Geometry check sheet. Reference: the model listing, model coordinates, mm. A direction names the side the tool comes from. Round coordinates to 2 decimals unless told otherwise and drop trailing zeros. Write each loop counter-clockwise with the first axis right and the second up, starting at its lowest first coordinate (ties: lowest second). Pieces come first, ordered by that corner, then holes. Notation, with made-up numbers: (-13.75, 58) -> (1.25, 58) arc R26 cw to (1.25, 81) -> close; hole circle Ø2 at (29, -35.5). An arc over 180 degrees is marked (long way). One line per question, with ' | ' between items.
Solid Edge part; units mm, degrees
sketch "Sketch1" plane through (0, 0, 0) normal (0, -1, 0) x (1, 0, 0)
  circle A0 centre (-17.5, 0) radius 1.6
  line L0 (-20.75, -18.3456) -> (-20.75, 0)
  line L1 (-9, -18.3456) -> (-20.75, -18.3456)
  line L2 (-9, -11.0482) -> (-9, -18.3456)
  arc A1 (-14.25, 0) -> (-9, -11.0482) centre (0, 0) ccw
  arc A2 (-20.75, 0) -> (-14.25, 0) centre (-17.5, 0) cw
  arc A3 (9, -11.0482) -> (14.25, 0) centre (0, 0) ccw
  arc A4 (14.25, 0) -> (20.75, 0) centre (17.5, 0) cw
  line L3 (20.75, 0) -> (20.75, -18.3456)
  line L4 (20.75, -18.3456) -> (9, -18.3456)
  line L5 (9, -18.3456) -> (9, -11.0482)
  circle A5 centre (17.5, 0) radius 1.6
  dimension "D1" = 17.5
extrude "Protrusion1" add sketch "Sketch1" against normal blind 6.5
sketch "Sketch2" plane through (14.875, 3.25, -18.3456) normal (0, 0, -1) x (0, -1, 0)
  line L0 (3.25, -5.875) -> (-25.75, -5.875)
  line L1 (-25.75, -5.875) -> (-25.75, 74.125)
  line L2 (-25.75, 74.125) -> (-5.75, 74.125)
  line L3 (-5.75, 74.125) -> (-5.75, 35.625)
  line L4 (-5.75, 35.625) -> (3.25, 35.625)
  line L5 (3.25, 35.625) -> (3.25, -5.875)
  dimension "D1" = 3.25
  dimension "D2" = 25.75
  dimension "D3" = 25.75
extrude "ExtrudedProtrusion_3" add sketch "Sketch2" along normal blind 10
sketch "Sketch3" plane through (-9.25, 14.5, -28.3456) normal (0, 0, -1) x (0, 1, 0)
  line L0 (-14.5, 12.25) -> (-14.5, 6.25)
  line L1 (-14.5, 6.25) -> (-10.5, 6.25)
  line L2 (-10.5, 6.25) -> (-10.5, 12.25)
  line L3 (-10.5, 12.25) -> (-14.5, 12.25)
  dimension "D1" = 10.5
  dimension "D2" = 10.5
extrude "ExtrudedCutout_1" cut sketch "Sketch3" against normal blind 42.3456
sketch "Sketch4" plane through (20.75, 14.5, -14.1728) normal (1, 0, 0) x (0, -1, 0)
  line L0 (-7, 4.1728) -> (8, -10.8272)
  line L1 (8, 4.1728) -> (8, -10.8272)
  line L2 (-7, 4.1728) -> (8, 4.1728)
extrude "Protrusion2" add sketch "Sketch4" against normal up to vertex (41.5 mm away)
sketch "Sketch5" plane through (-9.25, 19, -18.3456) normal (0, 0, 1) x (1, 0, 0)
  line L0 (-5, -12.5) -> (-5, 7.5538)
  line L1 (-5, 7.5538) -> (23.5, 7.5538)
  line L2 (23.5, 7.5538) -> (23.5, -12.5)
  line L3 (23.5, -12.5) -> (-5, -12.5)
extrude "ExtrudedCutout_2" cut sketch "Sketch5" along normal blind 49
sketch "Sketch6" plane through (-19.25, 14.5, -18.3456) normal (0, 0, 1) x (1, 0, 0)
  circle A0 centre (-35, 4.5) radius 1.6
  circle A1 centre (-15, 4.5) radius 1.6
extrude "ExtrudedCutout_3" cut sketch "Sketch6" against normal blind 30
chamfer "Letörés_1" distance 5 angle 45 11 edges at (-40, 9, -28.3456) (-40, 9, -18.3456) (-59.25, 9, -23.3456) (-59.25, 29, -23.3456) (-19.25, 29, -28.3456) (-19.25, 29, -18.3456) (20.75, 29, -23.3456) (20.75, 14.5, -28.3456) (-20.75, 4.5, -28.3456) (11.875, 0, -28.3456) (-11.875, 0, -28.3456)
chamfer "Letörés_3" distance 0.5 angle 45 9 edges at (-20.75, 14, -10.8456) (-14.25, 14, -10.8456) (14.25, 14, -10.8456) (20.75, 14, -10.8456) (20.75, 22.75, -18.3456) (-35.85, 19, -18.3456) (-35.85, 19, -28.3456) (-55.85, 19, -18.3456) (-55.85, 19, -28.3456)
chamfer "Letörés_4" distance 2 angle 45 4 edges at (-3, 0, -20.8456) (-3, 2, -25.3456) (3, 2, -25.3456) (3, 0, -20.8456)
(1) Sectioned sample at B-B on z = -15. Record the cut outline in (x, y).
Resolved:
outline: (-20.75, 0) -> (-9, 0) -> (-9, 6.5) -> (-14.25, 6.5) -> (-14.25, 17.45) -> (-14.75, 18.15) -> (-20.25, 18.15) -> (-20.75, 17.45) -> close; (9, 0) -> (20.75, 0) -> (20.75, 17.45) -> (20.25, 18.15) -> (14.75, 18.15) -> (14.25, 17.45) -> (14.25, 6.5) -> (9, 6.5) -> close
(2) Access from +Z, -Z, +X, -X, +Y, -Y to the whole of each face (thin tool, end or side, straight path). Record for faces 1 (the flat face through (-37.805, 11.535, -25.881)), 2 (the flat face through (-3, 3, -21)), 3 (the cylindrical face through (-12.908, 3.204, -6.036)), 4 (the flat face through (-13, 6.5, -8)).
Resolved:
face 1: -Z, -X, -Y | face 2: +Z, -Z, -Y | face 3: +Z, +Y, -Y | face 4: +Z, +Y
(3) Draft check along Z on faces 5 (the flat face through (-14, 17, -28.346)), 6 (the flat face through (-59.25, 19, -23)), 7 (the cylindrical face through (15.9, 3.2, 0.07)). Enter one of: +Z half, -Z half, draft (parallel to the pull), parting line (faces both ways), or undercut.
Resolved:
face 5: -Z half | face 6: draft | face 7: undercut
(4) Go/stop test with flat-tipped pins: pin 1 (1 mm diameter, centred on x = 4, y = 4.5, fed in from +Z); pin 2 (9.5 mm diameter, centred on x = -17.5, z = -5.5, fed in from +Y); pin 3 (4.5 mm diameter, centred on x = -1.5, z = -21, fed in from -Y); pin 4 (3 mm diameter, centred on x = -34.25, y = 19, fed in from +Z). Record where each tip stops, or that it passes through.
Resolved:
pin 1: stops at z = -18.35 | pin 2: stops at y = 13.4 | pin 3: stops at y = 1.25 | pin 4: passes through
(5) Sectioned sample at A-A on x = -34.25. Record the cut outline in (y, z).
Resolved:
outline: (9, -23.35) -> (14, -28.35) -> (16.9, -28.35) -> (17.4, -27.85) -> (17.4, -18.85) -> (16.9, -18.35) -> (14, -18.35) -> close; (20.6, -27.85) -> (21.1, -28.35) -> (24, -28.35) -> (29, -23.35) -> (24, -18.35) -> (21.1, -18.35) -> (20.6, -18.85) -> close
(6) Sectioned sample at C-C on y = 23. Record the cut outline in (x, z), then the cut area to 3 significant figures.
Resolved:
outline: (-59.25, -28.35) -> (15.75, -28.35) -> (20.75, -23.35) -> (20.75, -18.85) -> (20.25, -18.35) -> (-59.25, -18.35) -> close | area: 787 mm2
(7) Sectioned sample at D-D on x = -46.5. Record the cut outline in (y, z).
Resolved:
outline: (9, -23.35) -> (14, -28.35) -> (24, -28.35) -> (29, -23.35) -> (24, -18.35) -> (14, -18.35) -> close
(8) Material ranges on line 1 (X direction, y = 2.5, z = -17.5); line 2 (Z direction, x = 2, y = 23.5); line 3 (Z direction, x = -3, y = 24.5), recorded low to high.
Resolved:
line 1: x = -20.75 to -9, 9 to 20.75 | line 2: z = -28.35 to -18.35 | line 3: z = -27.85 to -18.85
